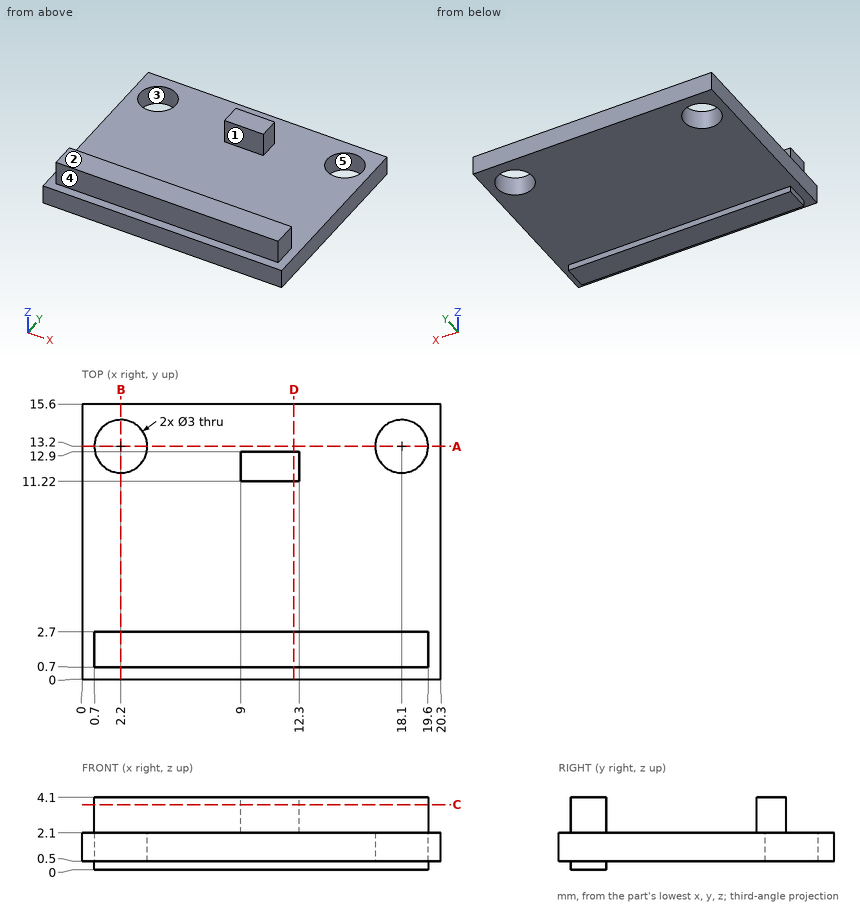
Input: dimensioned drawing with shaded views. Units: mm. Origin: part minimum x, y, z. A direction names the side the tool comes from. Coordinates: 2 decimals unless noted, no trailing zeros. Loops run counter-clockwise (first coordinate to the right, second up) from the corner with the lowest first, then second, coordinate; pieces in that order, holes last. Notation, with made-up numbers: (-36.5, 74) - (15.5, 74) arc R30 cw to (15.5, 110) - close; hole circle Ø9 at (62, 73). An arc over 180 degrees is marked (long way). One line per question, with ' | ' between items. Start each with the question number.
(1) First-contact query: pin 1 (1 mm diameter, centred on x = 10, z = 3, fed in from -Y); pin 2 (5 mm diameter, centred on x = 7.5, y = 6, fed in from +Z); pin 3 (1.6 mm diameter, centred on x = 12.5, z = 3, fed in from +Y). Flat tips, straight axial feed; report the tip coordinate or a pass-through.
(2) Ray query, L1, parallel to X at y = 13.2, z = 1.65; L2, parallel to Y at x = 18.1, z = 1.5; L3, parallel to Z at x = 12.75, y = 6.25. Return the intervals inside material, ascending. Write a range as from..to.
(3) Cut plane A-A on y = 13.2. Output: boundary loops of the cut face in (x, z).
(4) Reachability of the marked faces 1 and 2 from +Z, -Z, +X, -X, +Y, -Y: full face, straight path, thin tool, end or side. Return the list, or none.
(5) Cut plane B-B on x = 2.2. Output: boundary loops of the cut face in (y, z).
(6) Cut plane D-D on x = 12. Output: boundary loops of the cut face in (y, z), and give its area (3 significant figures).
(7) Cut plane C-C on z = 3.7. Output: boundary loops of the cut face in (x, y), and give its area (3 significant figures).
(8) Draft query along X for the marked faces 3, 4 and 5. Return one class per face: +X half, -X half, draft (parallel to the pull), parting line (faces both ways), or undercut.
Here are the results:
1) pin 1: y = 0.7 | pin 2: z = 2.1 | pin 3: y = 12.9
2) L1: 0..0.7, 3.7..16.6, 19.6..20.3 | L2: 0..11.7, 14.7..15.6 | L3: 0.5..2.1
3) outline: (0, 0.5) - (0.7, 0.5) - (0.7, 2.1) - (0, 2.1) - close; (3.7, 0.5) - (16.6, 0.5) - (16.6, 2.1) - (3.7, 2.1) - close; (19.6, 0.5) - (20.3, 0.5) - (20.3, 2.1) - (19.6, 2.1) - close
4) face 1: +Z, +X, -X | face 2: +Z, +X, -X, +Y, -Y
5) outline: (0, 0.5) - (0.7, 0.5) - (0.7, 0) - (2.7, 0) - (2.7, 0.5) - (11.7, 0.5) - (11.7, 2.1) - (2.7, 2.1) - (2.7, 4.1) - (0.7, 4.1) - (0.7, 2.1) - (0, 2.1) - close; (14.7, 0.5) - (15.6, 0.5) - (15.6, 2.1) - (14.7, 2.1) - close
6) outline: (0, 0.5) - (0.7, 0.5) - (0.7, 0) - (2.7, 0) - (2.7, 0.5) - (15.6, 0.5) - (15.6, 2.1) - (12.9, 2.1) - (12.9, 4.1) - (11.22, 4.1) - (11.22, 2.1) - (2.7, 2.1) - (2.7, 4.1) - (0.7, 4.1) - (0.7, 2.1) - (0, 2.1) - close | area: 33.3 mm²
7) outline: (0.7, 0.7) - (19.6, 0.7) - (19.6, 2.7) - (0.7, 2.7) - close; (9, 11.22) - (12.3, 11.22) - (12.3, 12.9) - (9, 12.9) - close | area: 43.3 mm²
8) face 3: undercut | face 4: draft | face 5: undercut
